Geometry check sheet. Reference: the model listing, model coordinates, mm. Give positions to 0.01 mm unless a question says otherwise; leave off trailing zeros. Order: outer loops, then holes, each group sorted by start corner. A loop starts at its lowest first (then second) coordinate and runs counter-clockwise, first axis right, second up.
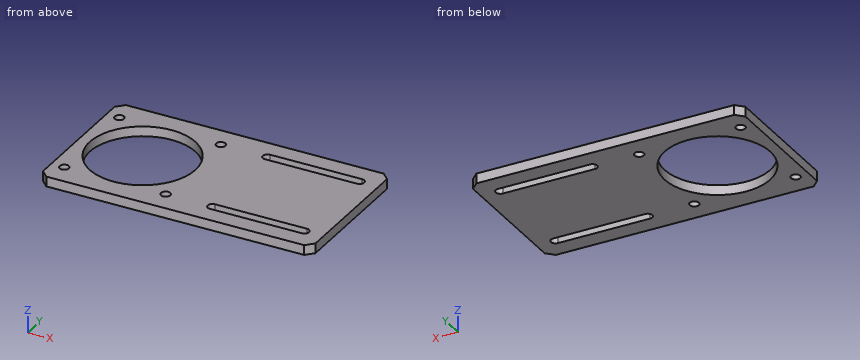
Autodesk Fusion 360 part; units mm, degrees
sketch "Sketch1" plane through (0, 0, 0) normal (0, 0, 1) x (1, 0, 0)
  line L0 (0, 0) -> (188, 0)
  line L1 (188, 0) -> (188, 101)
  line L2 (188, 101) -> (0, 101)
  line L3 (0, 101) -> (0, 0)
  circle A0 centre (44, 50.5) radius 36.5
  line L4 (0, 50.5) -> (188, 50.5) construction
  line L5 (9, 85.5) -> (79, 85.5) construction
  line L6 (79, 85.5) -> (79, 15.5) construction
  line L7 (79, 15.5) -> (9, 15.5) construction
  line L8 (9, 15.5) -> (9, 85.5) construction
  circle A1 centre (9, 85.5) radius 3.2
  circle A2 centre (79, 85.5) radius 3.2
  circle A3 centre (79, 15.5) radius 3.2
  circle A4 centre (9, 15.5) radius 3.2
  line L9 (111.2, 12.3) -> (174.8, 12.3)
  arc A5 (174.8, 12.3) -> (174.8, 18.7) centre (174.8, 15.5) ccw
  line L10 (174.8, 18.7) -> (111.2, 18.7)
  arc A6 (111.2, 18.7) -> (111.2, 12.3) centre (111.2, 15.5) ccw
  line L11 (111.2, 15.5) -> (174.8, 15.5) construction
  line L12 (111.2, 82.3) -> (174.8, 82.3)
  arc A7 (174.8, 82.3) -> (174.8, 88.7) centre (174.8, 85.5) ccw
  line L13 (174.8, 88.7) -> (111.2, 88.7)
  arc A8 (111.2, 88.7) -> (111.2, 82.3) centre (111.2, 85.5) ccw
  line L14 (111.2, 85.5) -> (174.8, 85.5) construction
  point P0 (44, 85.5)
  point P1 (9, 50.5)
  point P2 (178, 85.5)
  point P3 (108, 85.5)
  dimension "d1" = 188
  dimension "d2" = 101
  dimension "d3" = 73
  dimension "d4" = 70
  dimension "d5" = 6.4
  dimension "d6" = 9
  dimension "d7" = 10
  dimension "d8" = 70
extrude "Extrude1" add sketch "Sketch1" along normal blind 6.8
chamfer "Chamfer1" distance 5 angle 45 4 edges at (188, 101, 3.4) (188, 0, 3.4) (0, 0, 3.4) (0, 101, 3.4)
Q1. Thickness scan on L1, parallel to Y at x = 119.5, z = 1; L2, parallel to X at y = 13, z = 2; L3, parallel to Y at x = 44.5, z = 4.25. Record the ranges inside material, lowest first.
Q2. Cross-section at B-B, the plane z = 5.75. Record the boundary of the cut face in (x, y).
Q3. Cross-section at C-C, the plane x = 158. Record the boundary of the cut face in (y, z), and give its area (3 significant figures).
Q4. Gauge pin test, flat end, axial feed: P1, Ø4, axis at y = 81.5, z = 4, coming from the -X side. Record the tip position at first contact, or that the pin passes through.
Q5. Cross-section at A-A, the plane y = 50.5. Record the boundary of the cut face in (x, z), and give its area (3 significant figures).
Q6. Cross-section at D-D, the plane x = 71. Record the boundary of the cut face in (y, z), and give its area (3 significant figures).
Answers follow:
1. L1: y = 0 to 12.3, 18.7 to 82.3, 88.7 to 101
1. L2: x = 0 to 7, 11 to 77, 81 to 109.2, 176.8 to 188
1. L3: y = 0 to 14, 87 to 101
2. outline: (0, 5) - (5, 0) - (183, 0) - (188, 5) - (188, 96) - (183, 101) - (5, 101) - (0, 96) - close; hole circle Ø6.4 at (9, 15.5); hole circle Ø6.4 at (9, 85.5); hole circle Ø73 at (44, 50.5); hole circle Ø6.4 at (79, 15.5); hole circle Ø6.4 at (79, 85.5); hole (111.2, 12.3) - (174.8, 12.3) arc R3.2 ccw to (174.8, 18.7) - (111.2, 18.7) arc R3.2 ccw to start; hole (111.2, 82.3) - (174.8, 82.3) arc R3.2 ccw to (174.8, 88.7) - (111.2, 88.7) arc R3.2 ccw to start
3. outline: (0, 0) - (12.3, 0) - (12.3, 6.8) - (0, 6.8) - close; (18.7, 0) - (82.3, 0) - (82.3, 6.8) - (18.7, 6.8) - close; (88.7, 0) - (101, 0) - (101, 6.8) - (88.7, 6.8) - close
3. area: 600 mm2
4. P1: stops at x = 0
5. outline: (0, 0) - (7.5, 0) - (7.5, 6.8) - (0, 6.8) - close; (80.5, 0) - (188, 0) - (188, 6.8) - (80.5, 6.8) - close
5. area: 782 mm2
6. outline: (0, 0) - (25.94, 0) - (25.94, 6.8) - (0, 6.8) - close; (75.06, 0) - (101, 0) - (101, 6.8) - (75.06, 6.8) - close
6. area: 353 mm2
